Autodesk Inventor part; units mm, degrees
ref_plane "YZ Plane" through (0, 0, 0) normal (1, 0, 0) x (0, 1, 0)
ref_plane "XZ Plane" through (0, 0, 0) normal (0, 1, 0) x (-1, 0, 0)
ref_plane "XY Plane" through (0, 0, 0) normal (0, 0, 1) x (1, 0, 0)
sketch "Sketch1" plane through (0, 0, 0) normal (0, 0, 1) x (1, 0, 0)
  line L0 (0, 80) -> (0, 0)
  line L1 (0, 0) -> (70, 0)
  line L2 (70, 0) -> (70, 80)
  line L3 (6, 80) -> (6, 6)
  line L4 (6, 6) -> (64, 6)
  line L5 (64, 6) -> (64, 80)
  line L6 (0, 80) -> (6, 80)
  line L7 (64, 80) -> (70, 80)
  line L8 (0, -70) -> (70, -70)
  line L9 (0, -220) -> (0, -140)
  line L10 (0, -140) -> (70, -140)
  line L11 (70, -140) -> (70, -220)
  line L12 (6, -220) -> (6, -146)
  line L13 (6, -146) -> (64, -146)
  line L14 (64, -146) -> (64, -220)
  line L15 (0, -220) -> (6, -220)
  line L16 (64, -220) -> (70, -220)
  dimension "d0" = 70
  dimension "d1" = 80
  dimension "d2" = 80
  dimension "d3" = 6
  dimension "d10" = 70
extrude "Extrusion1" add sketch "Sketch1" along normal blind 50
sketch "Sketch2" plane through (0, 0, 0) normal (0, -1, 0) x (1, 0, 0)
  line L0 (6, 0) -> (0, 0)
  line L1 (0, 50) -> (70, 50)
  line L2 (0, 0) -> (70, 0)
  line L3 (70, 0) -> (70, 50)
  line L4 (70, 50) -> (0, 50)
  line L5 (0, 50) -> (0, 0)
  line L6 (6, 6) -> (64, 6)
  line L7 (64, 6) -> (64, 44)
  line L8 (64, 44) -> (6, 44)
  line L9 (6, 44) -> (6, 6)
  dimension "d7" = 6
extrude "Extrusion2" add sketch "Sketch2" along normal blind 140
properties part number "armj2"
For this review, take the finished solid that the model builds, in its own axes (mm). A direction names the side the tool comes from. Round coordinates to 2 decimals unless told otherwise and drop trailing zeros. Write each loop counter-clockwise with the first axis right and the second up, starting at its lowest first coordinate (ties: lowest second). Pieces come first, ordered by that corner, then holes. Notation, with made-up numbers: (-33.75, 59) - (21.25, 59) arc R14 ccw to (21.25, 73) - close; hole circle Ø2 at (73, -14.75). An arc over 180 degrees is marked (long way). Write each question's results on one line, items separated by ' | '.
Item 1: For faces 1 (the face through (6, -184, 25)), 2 (the face through (70, -68, 25)), 3 (the face through (35, -69, 6)), 4 (the face through (64, 42, 25)), list the 3-axis set-ups (+Z, -Z, +X, -X, +Y, -Y) from which the entire face can be reached by the end or side of a thin tool; tool diameter is ignored.
Calculated:
face 1: +Z, -Z, -Y | face 2: +Z, -Z, +X, +Y, -Y | face 3: none | face 4: +Z, -Z, +Y
Item 2: Take a section at A-A on y = -187.5. State the section outline as (x, z) points.
Calculated:
outline: (0, 0) - (6, 0) - (6, 50) - (0, 50) - close; (64, 0) - (70, 0) - (70, 50) - (64, 50) - close
Item 3: Take a section at B-B on z = 24. State the section outline as (x, y) points, then the cut area to 3 significant figures.
Calculated:
outline: (0, -220) - (6, -220) - (6, -146) - (64, -146) - (64, -220) - (70, -220) - (70, 80) - (64, 80) - (64, 6) - (6, 6) - (6, 80) - (0, 80) - close; hole (6, -140) - (64, -140) - (64, 0) - (6, 0) - close | area: 4,300 mm^2
Item 4: For pin 1 (1.5 mm diameter, centred on x = 11.5, z = 20.5, fed in from +Y); pin 2 (15 mm diameter, centred on x = 23.5, z = 33, fed in from -Y); pin 3 (3 mm diameter, centred on x = 59.5, y = -148.5, fed in from +Z), all flat-tipped, find the tip position at first contact; note any pin that passes through.
Calculated:
pin 1: stops at y = 6 | pin 2: stops at y = -146 | pin 3: passes through
Item 5: To check wall thickness, follow line 1 along Z through (x, y) = (25.5, -58); line 2 along X through (y, z) = (-189.5, 30.5); line 3 along Y through (x, z) = (54, 36.5). State the ranges of each line that lie inside material, in increasing order. Write a range as from..to.
Calculated:
line 1: z = 0..6, 44..50 | line 2: x = 0..6, 64..70 | line 3: y = -146..-140, 0..6
Item 6: Draft analysis for pull direction Z (two halves, no side actions). For faces 5 (the face through (64, -69, 25)), 6 (the face through (0, -68, 25)), 7 (the face through (35, -68, 0)), state which applies: pulls with the +Z half, pulls with the -Z half, needs draft (parallel to the pull), parting line crosses it, or undercut.
Calculated:
face 5: undercut | face 6: needs draft | face 7: pulls with the -Z half
Item 7: Take a section at C-C on y = -10.5. State the section outline as (x, z) points, then the cut area to 3 significant figures.
Calculated:
outline: (0, 0) - (70, 0) - (70, 50) - (0, 50) - close; hole (6, 6) - (64, 6) - (64, 44) - (6, 44) - close | area: 1,300 mm^2
Item 8: Take a section at D-D on x = 34. State the section outline as (y, z) points, then the cut area to 3 significant figures.
Calculated:
outline: (-146, 0) - (6, 0) - (6, 50) - (-146, 50) - close; hole (-140, 6) - (0, 6) - (0, 44) - (-140, 44) - close | area: 2,280 mm^2
